Answer from the drawing. Dimensions are ordinates in mm from the lowest x, y and z of the part. A direction names the side the tool comes from. Coordinates: 2 decimals unless noted, no trailing zeros. Write each loop counter-clockwise with the first axis right and the second up, starting at its lowest first coordinate (ties: lowest second). Pieces come first, ordered by that corner, then holes.
1) Find the intervals of material crossed by line 1 (Y direction, x = 120.5, z = 12.5); line 2 (X direction, y = 39, z = 34); line 3 (Z direction, x = 59.5, y = 36.5), in increasing order.
2) Which of the six approach directions +Z, -Z, +X, -X, +Y, -Y give full straight-line access (tool end or side, diameter ignored) to the marked faces 4 and 5?
3) The part is cut by section A-A (z = 38.5). Determine the outline of the cut face in (x, y).
4) The part is cut by section B-B (y = 23.5). Determine the outline of the cut face in (x, z), then the cut area to 3 significant figures.
5) Determine the mould class of the marked faces 1, 2 and 3 for opening direction X: +X half, -X half, draft (parallel to the pull), parting line (faces both ways), or undercut.
6) The part is cut by section C-C (x = 108). Determine the outline of the cut face in (y, z).
7) Each of these flat-tipped pins is pushed along its axis until it touches: pin 1 Ø10 at (x, y) = (67, 22.5) entering from -Z; pin 2 Ø12.5 at (y, z) = (34.5, 8.5) entering from +X; pin 3 Ø4 at (y, z) = (41.5, 24.5) entering from +X. Where does it stop, or does it pass through?
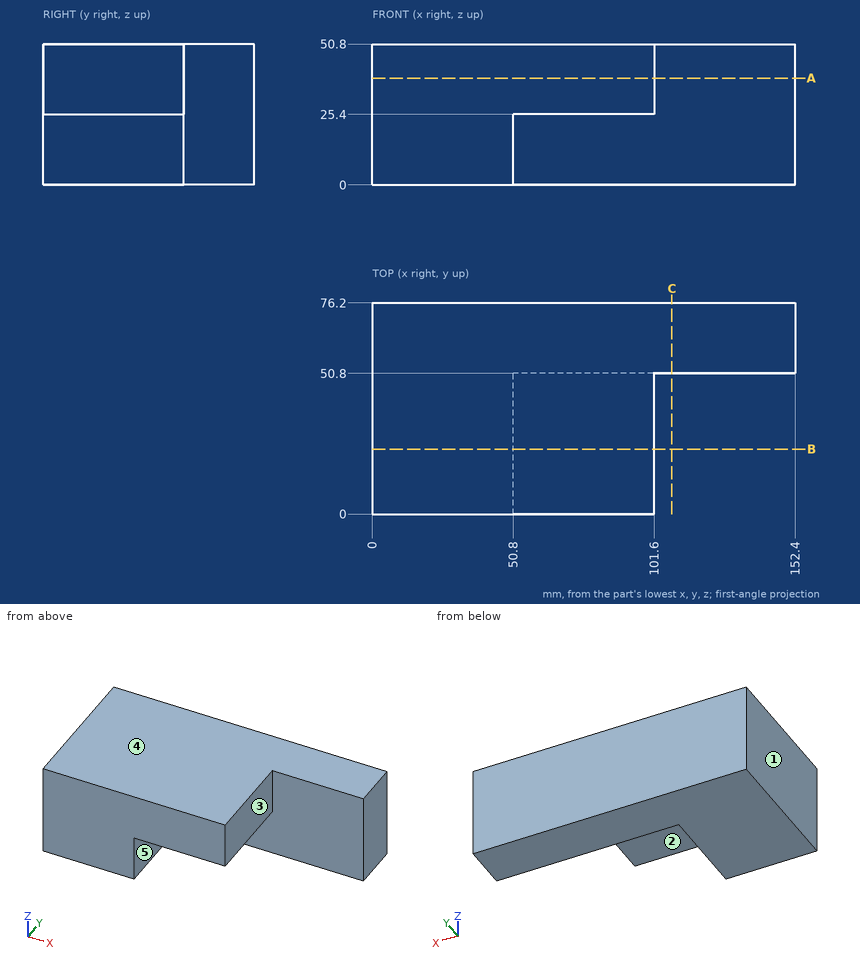
Reported:
1. line 1: y = 50.8 to 76.2
1. line 2: x = 0 to 101.6
1. line 3: z = 25.4 to 50.8
2. face 4: +Z, +X, -X, +Y, -Y
2. face 5: -Z, +X, -Y
3. outline: (0, 0) - (101.6, 0) - (101.6, 50.8) - (152.4, 50.8) - (152.4, 76.2) - (0, 76.2) - close
4. outline: (0, 0) - (50.8, 0) - (50.8, 25.4) - (101.6, 25.4) - (101.6, 50.8) - (0, 50.8) - close
4. area: 3,870 mm2
5. face 1: -X half
5. face 2: draft
5. face 3: +X half
6. outline: (50.8, 0) - (76.2, 0) - (76.2, 50.8) - (50.8, 50.8) - close
7. pin 1: stops at z = 25.4
7. pin 2: stops at x = 50.8
7. pin 3: stops at x = 101.6
